Geometry: final body of the model. Coordinates: model frame, mm. Round coordinates to 2 decimals unless told otherwise and drop trailing zeros. Order: outer loops, then holes, each group sorted by start corner. A loop starts at its lowest first (then second) coordinate and runs counter-clockwise, first axis right, second up. Notation, with made-up numbers: (65.25, -6.75) - (123.25, -6.75) arc R25 cw to (123.25, 29.25) - close; hole circle Ø8 at (4.5, 57). An arc over 180 degrees is marked (long way). Put each result on its own line as item: value. Start each with the question number.
(1) Section C-C (x = 16). Output: boundary loops of the cut face in (y, z), and give its area (3 significant figures).
(2) Section A-A (x = 62.5). Output: boundary loops of the cut face in (y, z), and give its area (3 significant figures).
(3) Pin query (flat end, axial travel): P1, Ø4, axis at x = 62.5, z = -24, coming from the -Y side. Return the tip coordinate at first contact, or that it passes through.
(4) Section B-B (y = 0.5). Output: boundary loops of the cut face in (x, z), and give its area (3 significant figures).
(5) Section D-D (z = -24). Output: boundary loops of the cut face in (x, y).
(6) Material intervals for L1, parallel to X at y = 0.95, z = -88; L2, parallel to X at y = 0.8, z = -24; L3, parallel to X at y = 0.75, z = -68, sorted ascending. Write a range as [from, to].
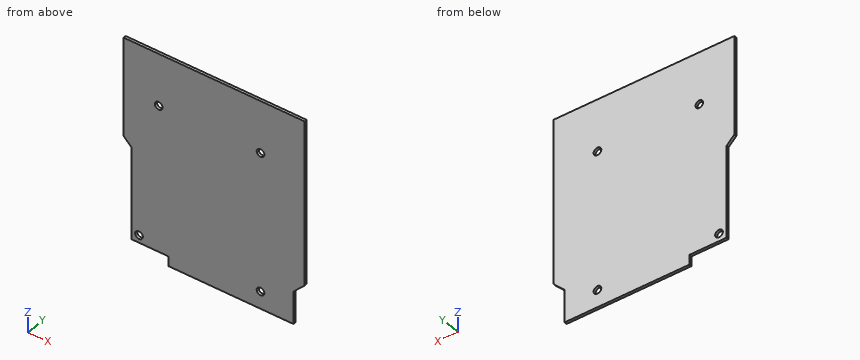
from build123d import *

# Parameters (mm, degrees)
SKETCH1_R = 1.75
PCB_DEPTH = 1.2


with BuildPart() as part:
    # Sketch1 → PCB (new body)
    with BuildSketch(Plane(origin=(0, 0, 0), x_dir=(1, 0, 0), z_dir=(0, 1, 0))):
        Polygon((0, 0), (0, 45.5), (3.5, 49), (3.5, 91.5), (20.5, 91.5), (20.5, 96), (77.5, 96), (77.5, 81), (82.5, 76), (82.5, 0), align=None)
        with Locations(Location((7, 88, 0), (0, 0, 270))):
            Circle(SKETCH1_R, mode=Mode.SUBTRACT)
        with Locations(Location((62.5, 88, 0), (0, 0, 270))):
            Circle(SKETCH1_R, mode=Mode.SUBTRACT)
        with Locations(Location((62.5, 24, 0), (0, 0, 270))):
            Circle(SKETCH1_R, mode=Mode.SUBTRACT)
        with Locations(Location((16, 24, 0), (0, 0, 270))):
            Circle(SKETCH1_R, mode=Mode.SUBTRACT)
    extrude(amount=PCB_DEPTH)


solid = part.part
Checks:
1. outline: (0, -91.5) - (1.2, -91.5) - (1.2, -25.75) - (0, -25.75) - close; (0, -22.25) - (1.2, -22.25) - (1.2, 0) - (0, 0) - close
1. area: 106 mm²
2. outline: (0, -96) - (1.2, -96) - (1.2, -89.75) - (0, -89.75) - close; (0, -86.25) - (1.2, -86.25) - (1.2, -25.75) - (0, -25.75) - close; (0, -22.25) - (1.2, -22.25) - (1.2, 0) - (0, 0) - close
2. area: 107 mm²
3. P1: stops at y = 0
4. outline: (0, -45.5) - (3.5, -49) - (3.5, -91.5) - (20.5, -91.5) - (20.5, -96) - (77.5, -96) - (77.5, -81) - (82.5, -76) - (82.5, 0) - (0, 0) - close; hole circle Ø3.5 at (7, -88); hole circle Ø3.5 at (16, -24); hole circle Ø3.5 at (62.5, -88); hole circle Ø3.5 at (62.5, -24)
4. area: 7,550 mm²
5. outline: (0, 0) - (14.25, 0) - (14.25, 1.2) - (0, 1.2) - close; (17.75, 0) - (60.75, 0) - (60.75, 1.2) - (17.75, 1.2) - close; (64.25, 0) - (82.5, 0) - (82.5, 1.2) - (64.25, 1.2) - close
6. L1: x = [3.5, 5.25], [8.75, 60.75], [64.25, 77.5]
6. L2: x = [0, 14.25], [17.75, 60.75], [64.25, 82.5]
6. L3: x = [3.5, 82.5]
